```python
from build123d import *

# Parameters (mm, degrees)
SKETCH1_W           = 5
SKETCH1_H           = 5
BOSS_EXTRUDE1_DEPTH = 110
SKETCH2_W           = 3
SKETCH2_H           = 3
CUT_EXTRUDE1_DEPTH  = 9
SKETCH3_W           = 3
SKETCH3_H           = 3
CUT_EXTRUDE2_DEPTH  = 9


with BuildPart() as part:
    # Sketch1 → Boss-Extrude1 (new body)
    with BuildSketch(Plane.XY):
        with Locations((2.5, 2.5)):
            Rectangle(SKETCH1_W, SKETCH1_H)
    extrude(amount=BOSS_EXTRUDE1_DEPTH)

    # Sketch2 → Cut-Extrude1 (cut)
    with BuildSketch(Plane.ZY):
        with Locations((2.5, 2.5)):
            Rectangle(SKETCH2_W, SKETCH2_H)
        with Locations((107.5, 2.5)):
            Rectangle(SKETCH2_W, SKETCH2_H)
        with Locations((13.5, 2.5)):
            Rectangle(SKETCH2_W, SKETCH2_H)
        with Locations((96.5, 2.5)):
            Rectangle(SKETCH2_W, SKETCH2_H)
    extrude(amount=-CUT_EXTRUDE1_DEPTH, mode=Mode.SUBTRACT)

    # Sketch3 → Cut-Extrude2 (cut)
    with BuildSketch(Plane(origin=(0, 5, 0), x_dir=(1, 0, 0), z_dir=(0, 1, 0))):
        with Locations((2.5, -25.15)):
            Rectangle(SKETCH3_W, SKETCH3_H)
        with Locations((2.5, -55)):
            Rectangle(SKETCH3_W, SKETCH3_H)
    extrude(amount=-CUT_EXTRUDE2_DEPTH, mode=Mode.SUBTRACT)


solid = part.part
```
Model file for the job. Use its own axes, mm. A direction names the side the tool comes from. Round coordinates to 2 decimals unless told otherwise and drop trailing zeros. Write each loop counter-clockwise with the first axis right and the second up, starting at its lowest first coordinate (ties: lowest second). Pieces come first, ordered by that corner, then holes. Notation, with made-up numbers: (-24.5, 78.25) - (-7.5, 78.25) arc R31 ccw to (-7.5, 105.25) - close; hole circle Ø3 at (13, 54). An arc over 180 degrees is marked (long way). Use CSV: the item, a comma, the result in double quotes. Start each with the question number.
Item 1: Tool access for faces 1 (the face through (2, 3, 0)), 2 (the face through (4, 3, 25)), 3 (the face through (2, 2, 106)): list every direction of +Z, -Z, +X, -X, +Y, -Y with a clear straight run to the whole face (end or side of a thin tool).
Item 2: Band-saw the part on B-B (z = 25.5). Write the cut outline in (x, y).
Item 3: Drill centre lines: L1, parallel to Z at x = 3.9, y = 4.65; L2, parallel to Z at x = 0.75, y = 1.05; L3, parallel to X at y = 0.95, z = 26.5. Where is each one in solid material? Low to high. Write a range as [from, to].
Item 4: Band-saw the part on A-A (y = 1.95). Write the cut outline in (x, z).
Item 5: Two-plate mould, pull along Y, no slides. Class faces 4 (the face through (2, 1, 107)), 5 (the face through (0.8, 5, 54.2)), 6 (the face through (2, 3, 23.65)), 7 (the face through (2, 2, 95)): released by +Y, released by -Y, zero draft, split by the parting line, or undercut.
Checked values:
1,face 1,"-Z, +X, -X, +Y, -Y"
1,face 2,"+Y, -Y"
1,face 3,"+X, -X"
2,outline,"(0, 0) - (1, 0) - (1, 5) - (0, 5) - close; (4, 0) - (5, 0) - (5, 5) - (4, 5) - close"
3,L1,"z = [0, 23.65], [26.65, 53.5], [56.5, 110]"
3,L2,"z = [0, 1], [4, 12], [15, 95], [98, 106], [109, 110]"
3,L3,"x = [0, 1], [4, 5]"
4,outline,"(0, 0) - (5, 0) - (5, 1) - (0, 1) - close; (0, 4) - (5, 4) - (5, 12) - (0, 12) - close; (0, 15) - (5, 15) - (5, 95) - (0, 95) - close; (0, 98) - (5, 98) - (5, 106) - (0, 106) - close; (0, 109) - (5, 109) - (5, 110) - (0, 110) - close; hole (1, 23.65) - (4, 23.65) - (4, 26.65) - (1, 26.65) - close; hole (1, 53.5) - (4, 53.5) - (4, 56.5) - (1, 56.5) - close"
5,face 4,"undercut"
5,face 5,"released by +Y"
5,face 6,"zero draft"
5,face 7,"undercut"
